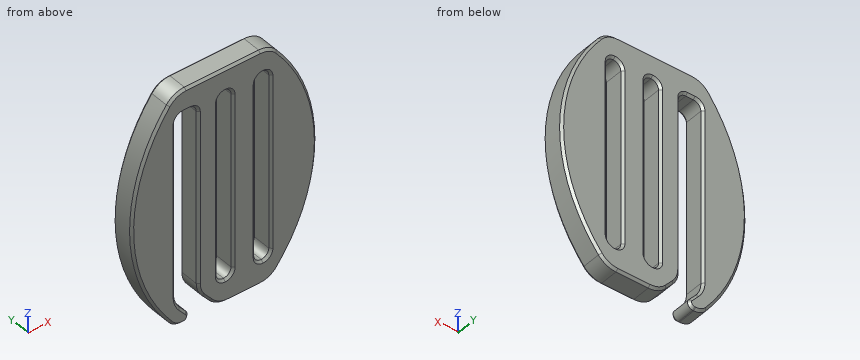
```python
from build123d import *

# Parameters (mm, degrees)
F1_DEPTH = 3
F2_SIZE  = 0.3


with BuildPart() as f1:
    # F0 (on Front) → F1 (new body)
    with BuildSketch(Plane.XZ):
        with BuildLine():
            ThreePointArc((8.6002542206, -4.5276246292), (9.6205467371, -5.289994744), (10.8651777768, -5.5603622459))
            Line((10.8651777768, -5.5603622459), (15.1357887981, -5.5603622459))
            ThreePointArc((15.1357887981, -5.5603622459), (16.4208285671, -5.2712058032), (17.4581499839, -4.4594774406))
            ThreePointArc((17.4581499839, -4.4594774406), (22.5960159615, 9.9396377541), (17.4581499839, 24.3387529488))
            ThreePointArc((17.4581499839, 24.3387529488), (16.4208285671, 25.1504813114), (15.1357887981, 25.4396377541))
            Line((15.1357887981, 25.4396377541), (9.4972672168, 25.4396377541))
            Line((9.4972672168, 25.4396377541), (5.3097819548, 25.4396377541))
            ThreePointArc((5.3097819548, 25.4396377541), (3.9825453513, 25.1300732205), (2.9292190014, 24.2652664198))
            ThreePointArc((2.9292190014, 24.2652664198), (-1.9299052308, 9.6676498918), (3.2652167583, -4.8137935487))
            ThreePointArc((3.2652167583, -4.8137935487), (3.9596707492, -5.3640893047), (4.8237128183, -5.5603622459))
            Line((4.8237128183, -5.5603622459), (4.9620791267, -5.5603622459))
            ThreePointArc((4.9620791267, -5.5603622459), (5.5989933763, -5.1507761552), (5.4905612898, -4.4013343565))
            Line((5.4905612898, -4.4013343565), (4.6266101762, -3.4066611267))
            ThreePointArc((4.6266101762, -3.4066611267), (4.0813050346, -2.4894533447), (3.8915337324, -1.4393987434))
            Line((3.8915337324, -1.4393987434), (3.8915337324, 21.4396377541))
            ThreePointArc((3.8915337324, 21.4396377541), (4.1844269512, 22.1467445353), (4.8915337324, 22.4396377541))
            Line((4.8915337324, 22.4396377541), (5.8915337324, 22.4396377541))
            ThreePointArc((5.8915337324, 22.4396377541), (6.5986405136, 22.1467445353), (6.8915337324, 21.4396377541))
            Line((6.8915337324, 21.4396377541), (6.8915337324, -1.4393987434))
            ThreePointArc((6.8915337324, -1.4393987434), (7.0813050346, -2.4894533447), (7.6266101762, -3.4066611267))
            Line((7.6266101762, -3.4066611267), (8.6002542206, -4.5276246292))
        make_face()
        with BuildLine():
            ThreePointArc((10.4972672168, 22.4396377541), (11.204373998, 22.1467445353), (11.4972672168, 21.4396377541))
            Line((11.4972672168, 21.4396377541), (11.4972672168, -1.5603622459))
            ThreePointArc((11.4972672168, -1.5603622459), (11.204373998, -2.2674690271), (10.4972672168, -2.5603622459))
            ThreePointArc((10.4972672168, -2.5603622459), (9.7901604356, -2.2674690271), (9.4972672168, -1.5603622459))
            Line((9.4972672168, -1.5603622459), (9.4972672168, 21.4396377541))
            ThreePointArc((9.4972672168, 21.4396377541), (9.7901604356, 22.1467445353), (10.4972672168, 22.4396377541))
        make_face(mode=Mode.SUBTRACT)
        with BuildLine():
            Line((14.4972672168, -1.5603622459), (14.4972672168, 21.4396377541))
            ThreePointArc((14.4972672168, 21.4396377541), (14.7901604356, 22.1467445353), (15.4972672168, 22.4396377541))
            ThreePointArc((15.4972672168, 22.4396377541), (16.204373998, 22.1467445353), (16.4972672168, 21.4396377541))
            Line((16.4972672168, 21.4396377541), (16.4972672168, -1.5603622459))
            ThreePointArc((16.4972672168, -1.5603622459), (16.204373998, -2.2674690271), (15.4972672168, -2.5603622459))
            ThreePointArc((15.4972672168, -2.5603622459), (14.7901604356, -2.2674690271), (14.4972672168, -1.5603622459))
        make_face(mode=Mode.SUBTRACT)
    extrude(amount=F1_DEPTH)

    # F2
    f2_edges = [f1.edges().sort_by_distance(p)[0] for p in [
        (4.081305, -3, -2.489453),
        (3.891534, -3, 10.00012),
        (4.184427, -3, 22.146745),
        (5.391534, -3, 22.439638),
        (6.598641, -3, 22.146745),
        (6.891534, -3, 10.00012),
        (7.081305, -3, -2.489453),
        (8.113432, -3, -3.967143),
        (9.620547, -3, -5.289995),
        (13.000483, -3, -5.560362),
        (16.420829, -3, -5.271206),
        (22.596016, -3, 9.939638),
        (16.420829, -3, 25.150481),
        (10.222785, -3, 25.439638),
        (3.982545, -3, 25.130073),
        (-1.929905, -3, 9.66765),
        (3.959671, -3, -5.364089),
        (4.892896, -3, -5.560362),
        (5.598993, -3, -5.150776),
        (5.058586, -3, -3.903998),
        (10.497267, -3, 22.439638),
        (11.497267, -3, 9.939638),
        (10.497267, -3, -2.560362),
        (9.497267, -3, 9.939638),
        (15.497267, -3, -2.560362),
        (14.497267, -3, 9.939638),
        (15.497267, -3, 22.439638),
        (16.497267, -3, 9.939638),
        (4.081305, 0, -2.489453),
        (3.891534, 0, 10.00012),
        (4.184427, 0, 22.146745),
        (5.391534, 0, 22.439638),
        (6.598641, 0, 22.146745),
        (6.891534, 0, 10.00012),
        (7.081305, 0, -2.489453),
        (8.113432, 0, -3.967143),
        (9.620547, 0, -5.289995),
        (13.000483, 0, -5.560362),
        (16.420829, 0, -5.271206),
        (22.596016, 0, 9.939638),
        (16.420829, 0, 25.150481),
        (10.222785, 0, 25.439638),
        (3.982545, 0, 25.130073),
        (-1.929905, 0, 9.66765),
        (3.959671, 0, -5.364089),
        (4.892896, 0, -5.560362),
        (5.598993, 0, -5.150776),
        (5.058586, 0, -3.903998),
        (10.497267, 0, 22.439638),
        (11.497267, 0, 9.939638),
        (10.497267, 0, -2.560362),
        (9.497267, 0, 9.939638),
        (15.497267, 0, -2.560362),
        (14.497267, 0, 9.939638),
        (15.497267, 0, 22.439638),
        (16.497267, 0, 9.939638),
    ]]
    chamfer(f2_edges, length=F2_SIZE)


solid = f1.part
```
Work out the finished part from the listing and answer in its coordinate system (mm). Give positions to 0.01 mm unless a question says otherwise; leave off trailing zeros. Loops run counter-clockwise (first coordinate to the right, second up) from the corner with the lowest first, then second, coordinate; pieces in that order, holes last. Notation, with made-up numbers: (-20.5, 22) -> (29.5, 22) arc R19 ccw to (29.5, 53) -> close; hole circle Ø5 at (68.25, 67). An arc over 180 degrees is marked (long way). Put each result on its own line as item: value. Start each with the question number.
Item 1: The part is cut by section B-B (z = 12). State how many separate pieces and enclosed holes the cut face has, then the cut area to 3 significant figures.
Item 2: Find the intervals of material crossed by L1, parallel to X at y = -1.45, z = 1.5; L2, parallel to X at y = -0.4, z = 19; L3, parallel to Z at x = 11, y = -2.4, in increasing order. Write a range as [from, to].
Item 3: The part is cut by section A-A (y = -1). Give the vertices of the cut face in (x, z), then the cut area to 3 significant figures.
Item 4: Each of these flat-tipped pins is pushed along its axis until it touches: P1, Ø1.2, axis at y = -1, z = 12, coming from the -X side; P2, Ø0.7, axis at y = -2, z = 4.5, coming from the +X side; P3, Ø6, axis at x = 4, z = 21.5, coming from the +Y side; P4, Ø0.8, axis at x = 5.5, y = -1.5, coming from the -Z side. Where does it stop, or does it pass through?
Answers below:
1. separate pieces: 4
1. enclosed holes: 0
1. area: 51.3 mm2
2. L1: [-0.37, 3.89], [6.89, 9.5], [11.5, 14.5], [16.5, 20.97]
2. L2: [-0.12, 3.89], [6.89, 9.5], [11.5, 14.5], [16.5, 20.71]
2. L3: [-5.56, -2.42], [22.3, 25.44]
3. outline: (2.93, 24.27) arc R23.54 ccw to (3.27, -4.81) arc R2 ccw to (4.82, -5.56) -> (4.96, -5.56) arc R0.7 ccw to (5.49, -4.4) -> (4.63, -3.41) arc R3 cw to (3.89, -1.44) -> (3.89, 21.44) arc R1 cw to (4.89, 22.44) -> (5.89, 22.44) arc R1 cw to (6.89, 21.44) -> (6.89, -1.44) arc R3 ccw to (7.63, -3.41) -> (8.6, -4.53) arc R3 ccw to (10.87, -5.56) -> (15.14, -5.56) arc R3 ccw to (17.46, -4.46) arc R22.75 ccw to (17.46, 24.34) arc R3 ccw to (15.14, 25.44) -> (5.31, 25.44) arc R3 ccw to start; hole (9.5, -1.56) arc R1 ccw to (11.5, -1.56) -> (11.5, 21.44) arc R1 ccw to (9.5, 21.44) -> close; hole (14.5, -1.56) arc R1 ccw to (16.5, -1.56) -> (16.5, 21.44) arc R1 ccw to (14.5, 21.44) -> close
3. area: 461 mm2
4. P1: x = -1.89
4. P2: x = 22.02
4. P3: y = 0
4. P4: z = -5.55
